Input: dimensioned drawing with shaded views. Units: mm. Origin: part minimum x, y, z. A direction names the side the tool comes from. Round coordinates to 2 decimals unless told otherwise and drop trailing zeros. Loops run counter-clockwise (first coordinate to the right, second up) from the corner with the lowest first, then second, coordinate; pieces in that order, holes last. Notation, with made-up numbers: M -19.75,26 L 32.25,26 A26 cw 32.25,55 Z; hole C -8.5,-38 d3. An arc over 180 degrees is marked long. Return JSON: item names as keys, results as strings.
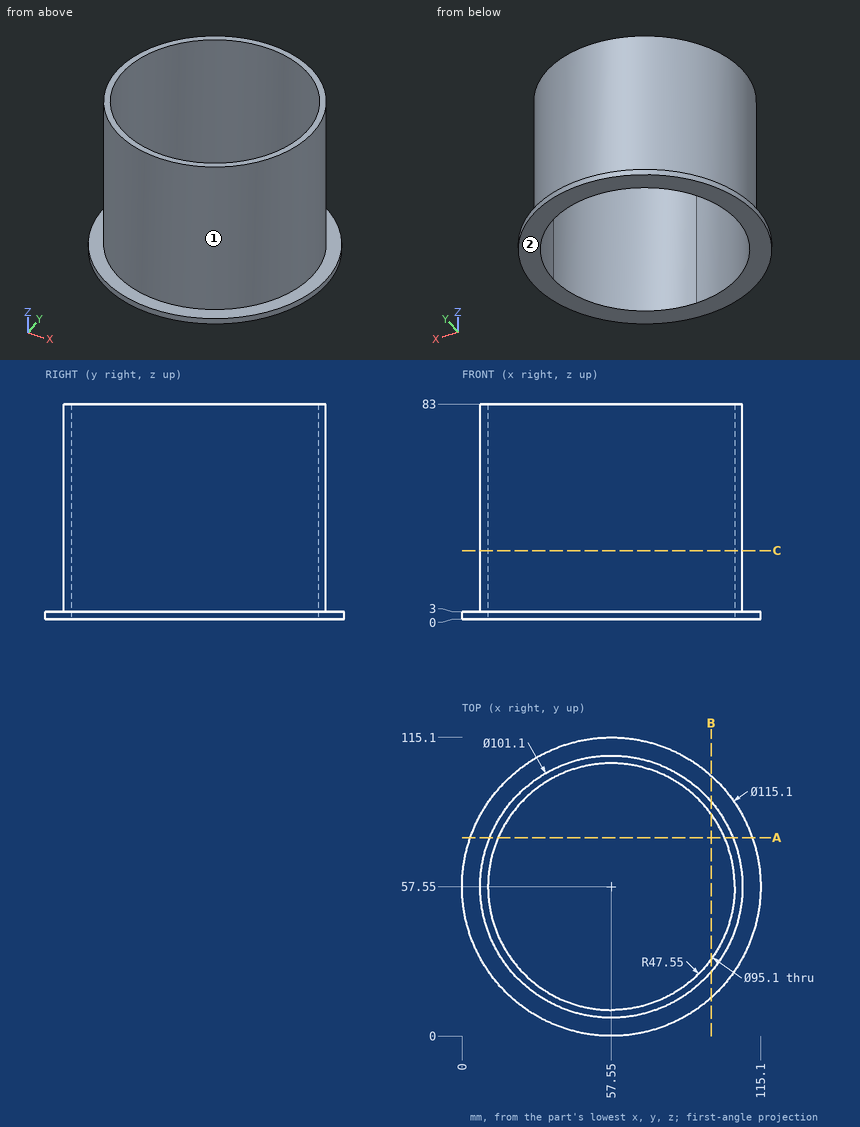
Q1. Section query C-C (z = 26.5). Output: boundary loops of the cut face in (x, y).
Determined:
{"outline": "C 57.55,57.55 d101.1; hole C 57.55,57.55 d95.1"}
Q2. Section query A-A (y = 76.5). Output: boundary loops of the cut face in (x, z), plus the area to 3 significant figures.
Determined:
{"outline": "M 3.21,0 L 13.94,0 L 13.94,83 L 10.69,83 L 10.69,3 L 3.21,3 Z; M 101.16,0 L 111.89,0 L 111.89,3 L 104.41,3 L 104.41,83 L 101.16,83 Z", "area": "585 mm^2"}
Q3. Reachability of the marked faces 1 and 2 from +Z, -Z, +X, -X, +Y, -Y: full face, straight path, thin tool, end or side. Return the list, or none.
Determined:
{"face 1": "+Z", "face 2": "-Z, +X, -X, +Y, -Y"}
Q4. Section query B-B (x = 96). Output: boundary loops of the cut face in (y, z), plus the area to 3 significant figures.
Determined:
{"outline": "M 14.73,0 L 29.58,0 L 29.58,83 L 24.73,83 L 24.73,3 L 14.73,3 Z; M 85.52,0 L 100.37,0 L 100.37,3 L 90.37,3 L 90.37,83 L 85.52,83 Z", "area": "864 mm^2"}
Q5. Pin query (flat end, axial travel): pin 1 (8 mm diameter, centred on x = 16.5, z = 18, fed in from -Y); pin 2 (2 mm diameter, centred on x = 42.5, z = 28, fed in from -Y); pin 3 (4 mm diameter, centred on x = 97, z = 38, fed in from +Y). Return the tip coordinate at first contact, or that it passes through.
Determined:
{"pin 1": "stops at y = 23.16", "pin 2": "stops at y = 8.99", "pin 3": "stops at y = 91.5"}
Q6. Material intervals for L1, parallel to X at y = 57.55, z = 34.5; L2, parallel to Y at x = 46.5, z = 14, sorted ascending.
Determined:
{"L1": "x = 7 to 10, 105.1 to 108.1", "L2": "y = 8.22 to 11.3, 103.8 to 106.88"}
